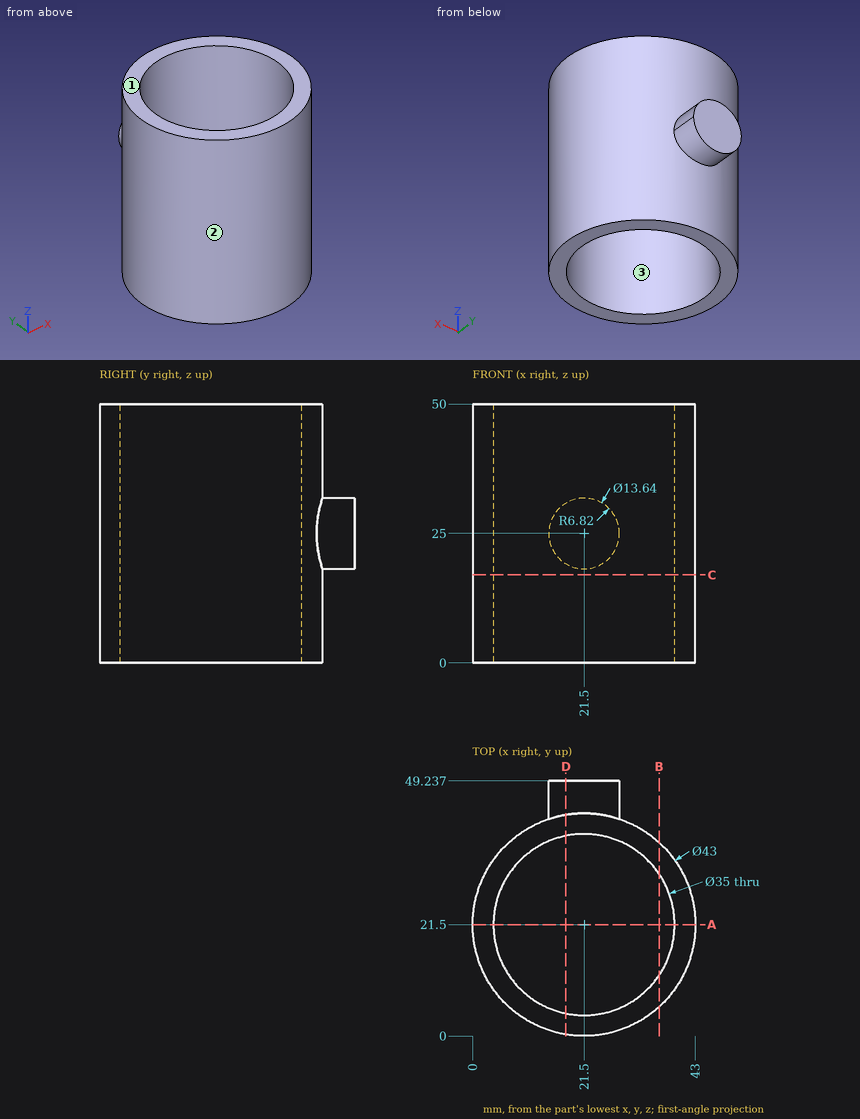
Verification items for this drawing (mm, ordinates from the low corner). Round coordinates to 2 decimals unless told otherwise and drop trailing zeros. Order: outer loops, then holes, each group sorted by start corner. A loop starts at its lowest first (then second) coordinate and runs counter-clockwise, first axis right, second up. Notation, with made-up numbers: (-35, 30) - (-10, 30) arc R13 ccw to (-10, 40) - close; hole circle Ø9 at (-8, 40.5). An arc over 180 degrees is marked (long way). Use CSV: the item, a comma, the result in double quotes.
(1) Thickness scan on probe 1 along Y at (x, z) = (21.5, 19.5); probe 2 along Y at (x, z) = (21.5, 39). Record the ranges inside material, lowest first. Write a range as from..to.
Entries:
probe 1,"0..4, 39..49.24"
probe 2,"0..4, 39..43"
(2) Section check B-B on x = 36. Record the boundary of the cut face in (y, z) (1 decimal).
Entries:
outline,"(5.6, 0) - (11.7, 0) - (11.7, 50) - (5.6, 50) - close; (31.3, 0) - (37.4, 0) - (37.4, 50) - (31.3, 50) - close"
(3) Section check C-C on z = 17. Record the boundary of the cut face in (x, y).
Entries:
outline,"circle Ø43 at (21.5, 21.5); hole circle Ø35 at (21.5, 21.5)"
(4) Mould release check, pull along X, two halves, no side actions. Record for the marked faces 1, 2 and 3: released by +X, released by -X, zero draft, split by the parting line, or undercut.
Entries:
face 1,"zero draft"
face 2,"split by the parting line"
face 3,"undercut"
(5) Gauge pin test, flat ends, axial feed: pin 1 Ø12 at (x, y) = (9, 20) entering from +Z; pin 2 Ø1 at (x, z) = (12.5, 18.5) entering from +Y; pin 3 Ø1.5 at (x, z) = (23.5, 20) entering from -Y; pin 4 Ø1 at (y, z) = (12.5, 38.5) entering from +X. Record the tip position at first contact, or that the pin passes through.
Entries:
pin 1,"z = 50"
pin 2,"y = 41.25"
pin 3,"y = 0.04"
pin 4,"x = 41.25"
(6) Section check A-A on y = 21.5. Record the boundary of the cut face in (x, z).
Entries:
outline,"(0, 0) - (4, 0) - (4, 50) - (0, 50) - close; (39, 0) - (43, 0) - (43, 50) - (39, 50) - close"
(7) Section check D-D on x = 18. Record the boundary of the cut face in (y, z).
Entries:
outline,"(0.29, 0) - (4.35, 0) - (4.35, 50) - (0.29, 50) - close; (38.65, 0) - (42.71, 0) - (42.71, 19.15) - (49.24, 19.15) - (49.24, 30.85) - (42.71, 30.85) - (42.71, 50) - (38.65, 50) - close"
